Read the model definition and answer for the solid it produces. Units are mm, in the model's axes. A direction names the side the tool comes from. Coordinates: 2 decimals unless noted, no trailing zeros. Write each loop counter-clockwise with the first axis right and the second up, starting at its lowest first coordinate (ties: lowest second). Pieces come first, ordered by that corner, then holes. Notation, with made-up numbers: (76, 14) -> (92, 14) arc R20 cw to (92, 49) -> close; hole circle Ø2 at (61, 69). An arc over 180 degrees is marked (long way). Answer in a Markdown table with one row per item. Add a question column.
Item 1: Section B-B on x = 21.5 is taken. Write down the section's boundary in (y, z).
Item 2: Given pin 1 Ø1.5 at (x, y) = (-6.5, 1) entering from -Z; pin 2 Ø0.9 at (x, y) = (-2, 1.5) entering from +Z; pin 3 Ø1.5 at (y, z) = (2, 20.5) entering from -X, each flat-ended and moving along its own axis, determine where each tip first touches the part or whether it passes through.
Item 3: Straight lines are drawn through the part: line 1 (Z direction, x = -19, y = 1.55); line 2 (X direction, y = 1.95, z = 10); line 3 (Z direction, x = -12.5, y = 2.05). For each, find the intervals that lie inside material, in ascending order. Write a range as from..to.
Item 4: Which of the six approach directions +Z, -Z, +X, -X, +Y, -Y give full straight-line access (tool end or side, diameter ignored) to faces 1 (the face through (1, 3, 11)), 2 (the face through (32.2, 2, -27))?
Item 5: Section A-A on y = 2.25 is taken. Count the separate pieces of the cut face and the enclosed holes in it, then the cut area to 3 significant figures.
Item 6: Section C-C on z = 10.5 is taken. Write down the section's boundary in (x, y).
Item 7: For a pull along X with two mould halves and no side action, classify faces 3 (the face through (1, 0, 11)), 4 (the face through (0, 2, 21.69)) as +X half, -X half, draft (parallel to the pull), parting line (faces both ways), or undercut.
Item 8: Section D-D on x = 7 is taken. Write down the section's boundary in (y, z).
```python
from build123d import *

# Parameters (mm, degrees)
SKETCH1_R           = 55
BOSS_EXTRUDE1_DEPTH = 3
CUT_EXTRUDE1_DEPTH  = 3
SKETCH4_R           = 1.5
SKETCH4_W           = 64.4
SKETCH4_H           = 3
CUT_EXTRUDE2_DEPTH  = 3


with BuildPart() as part:
    # Sketch1 → Boss-Extrude1 (new body)
    with BuildSketch(Plane(origin=(0, 0, 0), x_dir=(1, 0, 0), z_dir=(0, 1, 0))):
        with Locations(Location((0, 0, 0), (0, 0, 270))):
            Circle(SKETCH1_R)
    extrude(amount=BOSS_EXTRUDE1_DEPTH)

    # Sketch3 → Cut-Extrude1 (cut)
    with BuildSketch(Plane(origin=(0, 3, 0), x_dir=(1, 0, 0), z_dir=(0, 1, 0))):
        with BuildLine():
            Line((-25.359029713, 3.5), (0, 6.25))
            Line((0, 6.25), (25.359029713, 3.5))
            ThreePointArc((25.359029713, 3.5), (28.5, 0), (25.359029713, -3.5))
            Line((25.359029713, -3.5), (0, -6.25))
            Line((0, -6.25), (-25.359029713, -3.5))
            ThreePointArc((-25.359029713, -3.5), (-28.5, 0), (-25.359029713, 3.5))
        make_face()
    extrude(amount=-CUT_EXTRUDE1_DEPTH, mode=Mode.SUBTRACT)

    # Sketch4 → Cut-Extrude2 (cut)
    with BuildSketch(Plane(origin=(0, 3, 0), x_dir=(1, 0, 0), z_dir=(0, 1, 0))):
        with Locations(Location((-7, -10.5, 0), (0, 0, 270))):
            Circle(SKETCH4_R)
        with Locations(Location((7, -10.5, 0), (0, 0, 270))):
            Circle(SKETCH4_R)
        with Locations(Location((-7, 10.5, 0), (0, 0, 270))):
            Circle(SKETCH4_R)
        with Locations(Location((7, 10.5, 0), (0, 0, 270))):
            Circle(SKETCH4_R)
        with Locations((0, -20.19)):
            Rectangle(SKETCH4_W, SKETCH4_H)
        with Locations((0, -26.85)):
            Rectangle(SKETCH4_W, SKETCH4_H)
        with Locations((0, 26.84)):
            Rectangle(SKETCH4_W, SKETCH4_H)
    extrude(amount=-CUT_EXTRUDE2_DEPTH, mode=Mode.SUBTRACT)


solid = part.part
```
Results below:
| question | item | result |
|---|---|---|
| 1 | outline | (0, -50.62) -> (3, -50.62) -> (3, -28.34) -> (0, -28.34) -> close; (0, -25.34) -> (3, -25.34) -> (3, -3.92) -> (0, -3.92) -> close; (0, 3.92) -> (3, 3.92) -> (3, 18.69) -> (0, 18.69) -> close; (0, 21.69) -> (3, 21.69) -> (3, 25.35) -> (0, 25.35) -> close; (0, 28.35) -> (3, 28.35) -> (3, 50.62) -> (0, 50.62) -> close |
| 2 | pin 1 | stops at z = -54.7 |
| 2 | pin 2 | stops at z = 54.98 |
| 2 | pin 3 | stops at x = -51.33 |
| 3 | line 1 | z = -51.61..-28.34, -25.34..-4.19, 4.19..18.69, 21.69..25.35, 28.35..51.61 |
| 3 | line 2 | x = -54.08..-8.41, -5.59..5.59, 8.41..54.08 |
| 3 | line 3 | z = -53.56..-28.34, -25.34..-4.89, 4.89..18.69, 21.69..25.35, 28.35..53.56 |
| 4 | face 1 | +Z, -Z, +X, -X, +Y |
| 4 | face 2 | +Y, -Y |
| 5 | separate pieces | 1 |
| 5 | enclosed holes | 8 |
| 5 | area | 8,370 mm2 |
| 6 | outline | (-53.99, 0) -> (-8.5, 0) -> (-8.5, 3) -> (-53.99, 3) -> close; (-5.5, 0) -> (5.5, 0) -> (5.5, 3) -> (-5.5, 3) -> close; (8.5, 0) -> (53.99, 0) -> (53.99, 3) -> (8.5, 3) -> close |
| 7 | face 3 | draft |
| 7 | face 4 | undercut |
| 8 | outline | (0, -54.55) -> (3, -54.55) -> (3, -28.34) -> (0, -28.34) -> close; (0, -25.34) -> (3, -25.34) -> (3, -12) -> (0, -12) -> close; (0, -9) -> (3, -9) -> (3, -5.49) -> (0, -5.49) -> close; (0, 5.49) -> (3, 5.49) -> (3, 9) -> (0, 9) -> close; (0, 12) -> (3, 12) -> (3, 18.69) -> (0, 18.69) -> close; (0, 21.69) -> (3, 21.69) -> (3, 25.35) -> (0, 25.35) -> close; (0, 28.35) -> (3, 28.35) -> (3, 54.55) -> (0, 54.55) -> close |
